For this review, use the dimensioned drawing (mm, ordinates from the lowest corner) and the shaded views. Round coordinates to 2 decimals unless told otherwise and drop trailing zeros. Write each loop counter-clockwise with the first axis right and the second up, starting at its lowest first coordinate (ties: lowest second). Pieces come first, ordered by that corner, then holes. Notation, with made-up numbers: M -17,43.25 L 36,43.25 A31 ccw 36,70.25 Z; hole C 53.25,38.5 d5. An arc over 180 degrees is marked long. Answer in a Markdown table with one row per item.
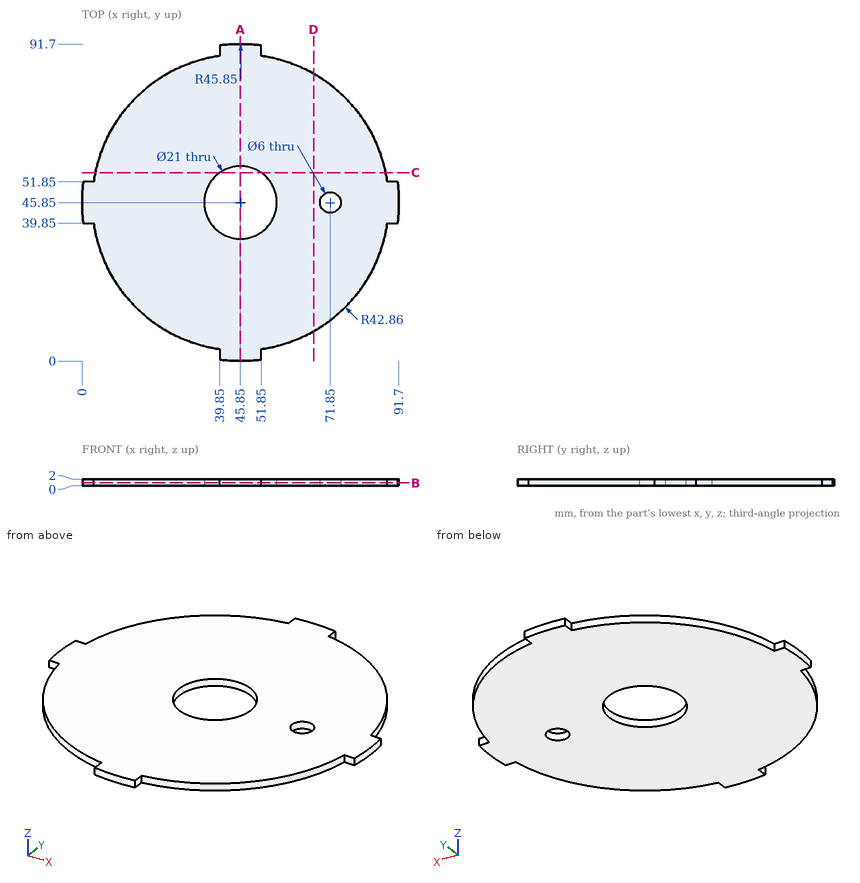
Q1. Take a section at B-B (z = 0.85). State the section outline as (x, y) points, then the cut area to 3 significant figures.
Found:
| item | result |
|---|---|
| outline | M 0.39,39.85 L 3.41,39.85 A42.86 ccw 39.85,3.41 L 39.85,0.39 A45.85 ccw 51.85,0.39 L 51.85,3.41 A42.86 ccw 88.29,39.85 L 91.31,39.85 A45.85 ccw 91.31,51.85 L 88.29,51.85 A42.86 ccw 51.85,88.29 L 51.85,91.31 A45.85 ccw 39.85,91.31 L 39.85,88.29 A42.86 ccw 3.41,51.85 L 0.39,51.85 A45.85 ccw Z; hole C 45.85,45.85 d21; hole C 71.85,45.85 d6 |
| area | 5,540 mm² |
Q2. Take a section at A-A (x = 45.85). State the section outline as (y, z) points, then the cut area to 3 significant figures.
Found:
| item | result |
|---|---|
| outline | M 0,0 L 35.35,0 L 35.35,2 L 0,2 Z; M 56.35,0 L 91.7,0 L 91.7,2 L 56.35,2 Z |
| area | 141 mm² |
Q3. Take a section at D-D (x = 67). State the section outline as (y, z) points.
Found:
| item | result |
|---|---|
| outline | M 8.57,0 L 83.13,0 L 83.13,2 L 8.57,2 Z |
Q4. For probe 1 along Y at (x, z) = (45.85, 1.4); probe 2 along X at (y, z) = (48, 0.4); probe 3 along X at (y, z) = (43.5, 0.7), list the stretches that pass through material, from the lowest coordinate up.
Found:
| item | result |
|---|---|
| probe 1 | 0 to 35.35, 56.35 to 91.7 |
| probe 2 | 0.05 to 35.57, 56.13 to 69.76, 73.94 to 91.65 |
| probe 3 | 0.06 to 35.62, 56.08 to 69.99, 73.71 to 91.64 |
Q5. Insertion check: P1, Ø0.6, axis at y = 1.5, z = 0.5, coming from the +X side; P2, Ø0.6, axis at x = 1.5, z = 1, coming from the +Y side; P3, Ø0.6, axis at y = 90, z = 1.5, coming from the -X side. Each pin has a flat end and moves straight along its axis. Give the tip position at first contact, or say it passes through.
Found:
| item | result |
|---|---|
| P1 | x = 51.85 |
| P2 | y = 51.85 |
| P3 | x = 39.85 |
Q6. Take a section at C-C (y = 54.5). State the section outline as (x, z) points.
Found:
| item | result |
|---|---|
| outline | M 3.87,0 L 39.9,0 L 39.9,2 L 3.87,2 Z; M 51.8,0 L 87.83,0 L 87.83,2 L 51.8,2 Z |
